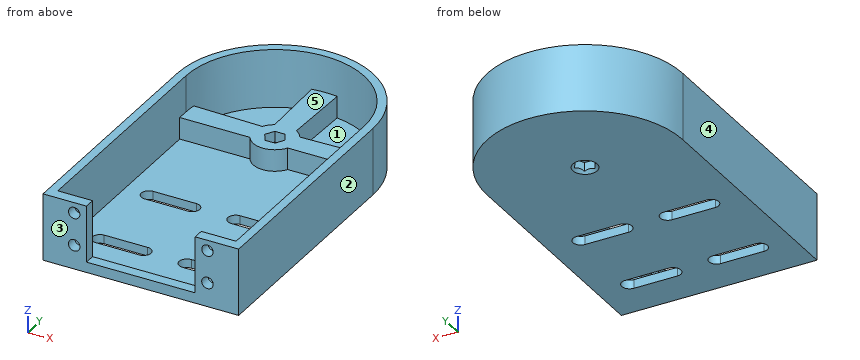
```python
from build123d import *

# Parameters (mm, degrees)
SALIENTE_EXTRUIR1_DEPTH                              = 4
CROQUIS2_R                                           = 2.75
SALIENTE_EXTRUIR2_DEPTH                              = 10
SALIENTE_EXTRUIR3_DEPTH                              = 30.8
CROQUIS4_R                                           = 2.75
CORTAR_EXTRUIR1_DEPTH                                = 4
REFRENTADO_PARA_TORNILLO_TAP_N_CON_CABEZ_D           = 5.5
REFRENTADO_PARA_TORNILLO_TAP_N_CON_CABEZ_CSINK_D     = 11.2
REFRENTADO_PARA_TORNILLO_TAP_N_CON_CABEZ_CSINK_ANGLE = 90
CORTAR_EXTRUIR2_DEPTH                                = 5
CORTAR_EXTRUIR3_DEPTH                                = 5
CORTAR_EXTRUIR4_DEPTH                                = 14
CROQUIS10_W                                          = 82
CROQUIS10_H                                          = 26.8
SALIENTE_EXTRUIR4_DEPTH                              = 5
CROQUIS11_R                                          = 2.619714774
CROQUIS11_W                                          = 50
CROQUIS11_H                                          = 26
CROQUIS11_R_2                                        = 2.655214408
CORTAR_EXTRUIR5_DEPTH                                = 5


with BuildPart() as part:
    # Croquis1 → Saliente-Extruir1 (new body)
    with BuildSketch(Plane.XY):
        with BuildLine():
            Line((-41, 0), (41, 0))
            Line((41, 0), (41, 110))
            ThreePointArc((41, 110), (0, 151), (-41, 110))
            Line((-41, 110), (-41, 0))
        make_face()
    extrude(amount=SALIENTE_EXTRUIR1_DEPTH)

    # Croquis2 → Saliente-Extruir2 (add)
    with BuildSketch(Plane.XY.offset(4)):
        with BuildLine():
            Line((-41, 105), (-8.660254038, 105))
            ThreePointArc((-8.660254038, 105), (0, 100), (8.660254038, 105))
            Line((8.660254038, 105), (41, 105))
            Line((41, 105), (41, 110))
            ThreePointArc((41, 110), (40.894733882, 112.936109791), (40.579476063, 115.857142857))
            Line((40.579476063, 115.857142857), (8.660254038, 115))
            ThreePointArc((8.660254038, 115), (7.071067812, 117.071067812), (5, 118.660254038))
            Line((5, 118.660254038), (5.857142857, 150.579476063))
            ThreePointArc((5.857142857, 150.579476063), (0, 151), (-5.857142857, 150.579476063))
            Line((-5.857142857, 150.579476063), (-5, 118.660254038))
            ThreePointArc((-5, 118.660254038), (-7.071067812, 117.071067812), (-8.660254038, 115))
            Line((-8.660254038, 115), (-40.579476063, 115.857142857))
            ThreePointArc((-40.579476063, 115.857142857), (-40.894733882, 112.936109791), (-41, 110))
            Line((-41, 110), (-41, 105))
        make_face()
        with Locations((0, 110)):
            Circle(CROQUIS2_R, mode=Mode.SUBTRACT)
    extrude(amount=SALIENTE_EXTRUIR2_DEPTH)

    # Croquis3 → Saliente-Extruir3 (add)
    with BuildSketch(Plane(origin=(0, 0, 0), x_dir=(-1, 0, 0), z_dir=(0, 0, -1))):
        with BuildLine():
            Line((-41, 0), (-41, 110))
            ThreePointArc((-41, 110), (0, 151), (41, 110))
            Line((41, 110), (41, 0))
            Line((41, 0), (45, 0))
            Line((45, 0), (45, 110))
            ThreePointArc((45, 110), (0, 155), (-45, 110))
            Line((-45, 110), (-45, 0))
            Line((-45, 0), (-41, 0))
        make_face()
    extrude(amount=-SALIENTE_EXTRUIR3_DEPTH)

    # Croquis4 → Cortar-Extruir1 (cut)
    with BuildSketch(Plane.XY.offset(4)):
        with Locations((0, 110)):
            Circle(CROQUIS4_R)
    extrude(amount=-CORTAR_EXTRUIR1_DEPTH, mode=Mode.SUBTRACT)

    # Refrentado para tornillo tapón con cabeza plana de clavija de M52 (through all)
    with Locations(Plane(origin=(0, 110, 0), x_dir=(-1, 0, 0), z_dir=(0, 0, -1))):
        with Locations((0, 0)):
            CounterSinkHole(REFRENTADO_PARA_TORNILLO_TAP_N_CON_CABEZ_D / 2, REFRENTADO_PARA_TORNILLO_TAP_N_CON_CABEZ_CSINK_D / 2, counter_sink_angle=REFRENTADO_PARA_TORNILLO_TAP_N_CON_CABEZ_CSINK_ANGLE)

    # Croquis7 → Cortar-Extruir2 (cut)
    with BuildSketch(Plane(origin=(0, 0, 0), x_dir=(-1, 0, 0), z_dir=(0, 0, -1))):
        Polygon((2.189291013, 105.834926388), (4.701705063, 109.813444827), (2.512414051, 113.978518439), (-2.189291013, 114.165073612), (-4.701705063, 110.186555173), (-2.512414051, 106.021481561), align=None)
    extrude(amount=-CORTAR_EXTRUIR2_DEPTH, mode=Mode.SUBTRACT)

    # Croquis8 → Cortar-Extruir3 (cut)
    with BuildSketch(Plane.XY.offset(14)):
        Polygon((4.705404694, 110), (2.352702347, 114.075), (-2.352702347, 114.075), (-4.705404694, 110), (-2.352702347, 105.925), (2.352702347, 105.925), align=None)
    extrude(amount=-CORTAR_EXTRUIR3_DEPTH, mode=Mode.SUBTRACT)

    # Croquis9 → Cortar-Extruir4 (cut)
    with BuildSketch(Plane.XY.offset(14)):
        with BuildLine():
            Line((-30, 63.448836188), (-10, 63.448836188))
            ThreePointArc((-10, 63.448836188), (-6.551163812, 60), (-10, 56.551163812))
            Line((-10, 56.551163812), (-30, 56.551163812))
            ThreePointArc((-30, 56.551163812), (-33.448836188, 60), (-30, 63.448836188))
        make_face()
        with BuildLine():
            Line((10, 63.580626855), (30, 63.580626855))
            ThreePointArc((30, 63.580626855), (33.580626855, 60), (30, 56.419373145))
            Line((30, 56.419373145), (10, 56.419373145))
            ThreePointArc((10, 56.419373145), (6.419373145, 60), (10, 63.580626855))
        make_face()
        with BuildLine():
            Line((-30, 16.551163812), (-10, 16.551163812))
            ThreePointArc((-10, 16.551163812), (-6.551163812, 20), (-10, 23.448836188))
            Line((-10, 23.448836188), (-30, 23.448836188))
            ThreePointArc((-30, 23.448836188), (-33.448836188, 20), (-30, 16.551163812))
        make_face()
        with BuildLine():
            Line((10, 16.419373145), (30, 16.419373145))
            ThreePointArc((30, 16.419373145), (33.580626855, 20), (30, 23.580626855))
            Line((30, 23.580626855), (10, 23.580626855))
            ThreePointArc((10, 23.580626855), (6.419373145, 20), (10, 16.419373145))
        make_face()
    extrude(amount=-CORTAR_EXTRUIR4_DEPTH, mode=Mode.SUBTRACT)

    # Croquis10 → Saliente-Extruir4 (add)
    with BuildSketch(Plane(origin=(0, 5, 0), x_dir=(-1, 0, 0), z_dir=(0, -1, 0))):
        with Locations((0, -17.4)):
            Rectangle(CROQUIS10_W, CROQUIS10_H)
    extrude(amount=SALIENTE_EXTRUIR4_DEPTH)

    # Croquis11 → Cortar-Extruir5 (cut)
    with BuildSketch(Plane.XZ):
        with Locations((-30.65, 26)):
            Circle(CROQUIS11_R)
        with Locations((0, 17.8)):
            Rectangle(CROQUIS11_W, CROQUIS11_H)
        with Locations((30.65, 26)):
            Circle(CROQUIS11_R)
        with Locations((30.65, 11)):
            Circle(CROQUIS11_R_2)
        with Locations((-30.65, 11)):
            Circle(CROQUIS11_R_2)
    extrude(amount=-CORTAR_EXTRUIR5_DEPTH, mode=Mode.SUBTRACT)


solid = part.part
```
Part model, mm, in its own coordinate system. Face numbers are marked on the shaded views. A direction names the side the tool comes from. Round coordinates to 2 decimals unless told otherwise and drop trailing zeros. Loops run counter-clockwise (first coordinate to the right, second up) from the corner with the lowest first, then second, coordinate; pieces in that order, holes last.
Item 1: Cut at B-B, the plane x = 0. Give the cut face in (y, z) (3 decimals).
Item 2: Cut at A-A, the plane z = 26. Give the cut face in (x, y).
Item 3: Cut at D-D, the plane y = 83. Give the cut face in (x, z), then the cut area to 3 significant figures.
Item 4: Drop flat-ended pins along their axis: P1, Ø5, axis at x = -5, z = 9.5, coming from the -Y side; P2, Ø8, axis at x = 10, z = 20, coming from the +Y side; P3, Ø4, axis at x = -28.5, y = 109.5, coming from the +Z side. Give the stop position or say it passes through.
Item 5: Mould opens along Y. For the marked faces 3, 4 and 5 say: +Y half, -Y half, draft (parallel to the pull), parting line (faces both ways), or undercut.
Item 6: Cut at C-C, the plane y = 60. Give the cut face in (x, z), then the cut area to 3 significant figures.
Item 7: Drill centre lines: line 1 (Z direction, x = 30.65, y = 3.2); line 2 (X direction, y = 83, z = 21.5); line 3 (Z direction, x = -30, y = 3). Where is each one in solid material? Low to high.
Item 8: 3-axis set-ups, long thin cutter, end or side, ignore diameter. For the marked faces 1 and 2: which of +Z, -Z, +X, -X, +Y, -Y reach the whole face in a straight line?
A:
1. outline: (0, 0) - (104.4, 0) - (105.922, 1.522) - (105.922, 5) - (107.25, 5) - (107.25, 9) - (105.925, 9) - (105.925, 14) - (100, 14) - (100, 4) - (5, 4) - (5, 4.8) - (0, 4.8) - close; (112.75, 5) - (114.078, 5) - (114.078, 1.522) - (115.6, 0) - (155, 0) - (155, 30.8) - (151, 30.8) - (151, 14) - (114.075, 14) - (114.075, 9) - (112.75, 9) - close
2. outline: (-45, 0) - (-33.27, 0) - (-33.27, 5) - (-41, 5) - (-41, 110) arc R41 cw to (41, 110) - (41, 5) - (33.27, 5) - (33.27, 0) - (45, 0) - (45, 110) arc R45 ccw to (-45, 110) - close; (-28.03, 0) - (-25, 0) - (-25, 5) - (-28.03, 5) - close; (25, 0) - (28.03, 0) - (28.03, 5) - (25, 5) - close
3. outline: (-45, 0) - (45, 0) - (45, 30.8) - (41, 30.8) - (41, 4) - (-41, 4) - (-41, 30.8) - (-45, 30.8) - close
3. area: 574 mm2
4. P1: stops at y = 100.32
4. P2: stops at y = 154.6
4. P3: stops at z = 14
5. face 3: -Y half
5. face 4: draft
5. face 5: undercut
6. outline: (-45, 0) - (-33.45, 0) - (-33.45, 4) - (-41, 4) - (-41, 30.8) - (-45, 30.8) - close; (-6.55, 0) - (6.42, 0) - (6.42, 4) - (-6.55, 4) - close; (33.58, 0) - (45, 0) - (45, 30.8) - (41, 30.8) - (41, 4) - (33.58, 4) - close
6. area: 358 mm2
7. line 1: z = 0 to 8.34, 13.66 to 23.38, 28.62 to 30.8
7. line 2: x = -45 to -41, 41 to 45
7. line 3: z = 0 to 8.43, 13.57 to 23.46, 28.54 to 30.8
8. face 1: +Z
8. face 2: +Z, -Z, +X, +Y, -Y
